from build123d import *

# Parameters (mm, degrees)
SKETCH1_W           = 60
SKETCH1_H           = 180
SKETCH1_W_2         = 180
SKETCH1_H_2         = 60
BOSS_EXTRUDE1_DEPTH = 10
SKETCH2_R           = 4.5
CUT_EXTRUDE1_DEPTH  = 11


with BuildPart() as part:
    # Sketch1 → Boss-Extrude1 (new body)
    with BuildSketch(Plane(origin=(0, 0, 0), x_dir=(1, 0, 0), z_dir=(0, 1, 0))):
        with Locations((-120, 0)):
            Rectangle(SKETCH1_W, SKETCH1_H)
        Polygon((-90, -90), (-150, -90), (-90, -150), align=None)
        Polygon((-90, 90), (-90, 150), (-150, 90), align=None)
        with Locations((0, 120)):
            Rectangle(SKETCH1_W_2, SKETCH1_H_2)
        Rectangle(SKETCH1_W_2, SKETCH1_H)
        with Locations((0, -120)):
            Rectangle(SKETCH1_W_2, SKETCH1_H_2)
        Polygon((150, -90), (90, -90), (90, -150), align=None)
        with Locations((120, 0)):
            Rectangle(SKETCH1_W, SKETCH1_H)
        Polygon((150, 90), (90, 150), (90, 90), align=None)
    extrude(amount=BOSS_EXTRUDE1_DEPTH)

    # Sketch2 → Cut-Extrude1 (cut, through all)
    with BuildSketch(Plane(origin=(0, 10, 0), x_dir=(1, 0, 0), z_dir=(0, 1, 0))):
        with Locations((-78, 140)):
            Circle(SKETCH2_R)
        with Locations((-140, 78)):
            Circle(SKETCH2_R)
        with Locations((-140, -78)):
            Circle(SKETCH2_R)
        with Locations((-78, -140)):
            Circle(SKETCH2_R)
        with Locations((78, -140)):
            Circle(SKETCH2_R)
        with Locations((140, -78)):
            Circle(SKETCH2_R)
        with Locations((140, 78)):
            Circle(SKETCH2_R)
        with Locations((78, 140)):
            Circle(SKETCH2_R)
    extrude(amount=-CUT_EXTRUDE1_DEPTH, mode=Mode.SUBTRACT)


solid = part.part
Check sheet for the modelled part. Datum: model origin and axes. Units: mm. Round coordinates to 2 decimals unless told otherwise and drop trailing zeros. Order: outer loops, then holes, each group sorted by start corner. A loop starts at its lowest first (then second) coordinate and runs counter-clockwise, first axis right, second up.
(1) Cross-section at D-D, the plane x = -127.5. Enter the section's corners in (y, z).
(2) Cross-section at A-A, the plane x = 78. Enter the section's corners in (y, z), and give its area (3 significant figures).
(3) Cross-section at B-B, the plane z = -78. Enter the section's corners in (x, y), and give its area (3 significant figures).
(4) Scan lines: probe 1 along Z at (x, y) = (-78, 5.75); probe 2 along X at (y, z) = (6.5, -140). Record each from-to range of solid material in increasing order.
(5) Go/stop test with a flat-tipped pin: P1, Ø7, axis at x = 140, z = 78, coming from the -Y side. Record where the tip stops, or that it passes through.
(6) Draft check along X on faces 1 (the cylindrical face through (-78.98, 5.07, 144.39)), 2 (the flat face through (-120, 5, -120)), 3 (the flat face through (150, 5, 1)). Enter one of: pulls with the +X half, pulls with the -X half, needs draft (parallel to the pull), parting line crosses it, or undercut.
(7) Cross-section at C-C, the plane y = 4. State how many separate pieces and enclosed holes the cut face has, and give its area (3 significant figures).
Check sheet entries:
1. outline: (0, -112.5) - (10, -112.5) - (10, 112.5) - (0, 112.5) - close
2. outline: (0, -150) - (10, -150) - (10, -144.5) - (0, -144.5) - close; (0, -135.5) - (10, -135.5) - (10, 135.5) - (0, 135.5) - close; (0, 144.5) - (10, 144.5) - (10, 150) - (0, 150) - close
2. area: 2,820 mm2
3. outline: (-150, 0) - (-144.5, 0) - (-144.5, 10) - (-150, 10) - close; (-135.5, 0) - (135.5, 0) - (135.5, 10) - (-135.5, 10) - close; (144.5, 0) - (150, 0) - (150, 10) - (144.5, 10) - close
3. area: 2,820 mm2
4. probe 1: z = -150 to -144.5, -135.5 to 135.5, 144.5 to 150
4. probe 2: x = -100 to -82.5, -73.5 to 73.5, 82.5 to 100
5. P1: passes through
6. face 1: undercut
6. face 2: pulls with the -X half
6. face 3: pulls with the +X half
7. separate pieces: 1
7. enclosed holes: 8
7. area: 82,300 mm2
